Model file for the job. Use its own axes, mm. Round coordinates to 2 decimals unless told otherwise and drop trailing zeros. Write each loop counter-clockwise with the first axis right and the second up, starting at its lowest first coordinate (ties: lowest second). Pieces come first, ordered by that corner, then holes. Notation, with made-up numbers: (1, 69.5) - (13, 69.5) arc R23 ccw to (13, 102.5) - close; hole circle Ø1 at (-11, 43). An arc over 180 degrees is marked (long way). One line per item, written item: value.
Autodesk Inventor part; units mm, degrees
ref_plane "YZ Plane" through (0, 0, 0) normal (1, 0, 0) x (0, 1, 0)
ref_plane "XZ Plane" through (0, 0, 0) normal (0, 1, 0) x (-1, 0, 0)
ref_plane "XY Plane" through (0, 0, 0) normal (0, 0, 1) x (1, 0, 0)
sketch "Sketch1" plane through (0, 0, 0) normal (0, 1, 0) x (-1, 0, 0)
  line L0 (3.175, 0) -> (9.525, 0)
  line L1 (12.7, 3.175) -> (12.7, 200.025)
  line L2 (9.525, 203.2) -> (3.175, 203.2)
  line L3 (0, 200.025) -> (0, 3.175)
  circle A0 centre (6.35, 6.35) radius 2.5797
  circle A1 centre (6.35, 196.85) radius 2.5797
  circle A2 centre (6.35, 101.6) radius 2.5797
  arc A3 (12.7, 200.025) -> (9.525, 203.2) centre (9.525, 200.025) ccw
  arc A4 (3.175, 203.2) -> (0, 200.025) centre (3.175, 200.025) ccw
  arc A5 (0, 3.175) -> (3.175, 0) centre (3.175, 3.175) ccw
  arc A6 (9.525, 0) -> (12.7, 3.175) centre (9.525, 3.175) ccw
  point P0 (0, 0)
  point P1 (12.7, 0)
  point P2 (0, 203.2)
  dimension "d0" = 203.2
  dimension "d1" = 12.7
  dimension "d2" = 5.1594
  dimension "d3" = 6.35
  dimension "d4" = 6.35
  dimension "d5" = 5.1594
  dimension "d6" = 6.35
  dimension "d7" = 6.35
  dimension "d8" = 6.35
  dimension "d9" = 5.1594
  dimension "d10" = 101.6
  dimension "d11" = 3.175
extrude "Extrusion1" add sketch "Sketch1" along normal blind 9.525
fillet "Fillet1" radius 3.175 16 edges at (-0.9299, 9.525, 0.9299) (-6.35, 9.525, 0) (-11.7701, 9.525, 0.9299) (-12.7, 9.525, 101.6) (-11.7701, 9.525, 202.2701) (-6.35, 9.525, 203.2) (-0.9299, 9.525, 202.2701) (0, 9.525, 101.6) (-0.9299, 0, 0.9299) (-6.35, 0, 0) (-11.7701, 0, 0.9299) (-12.7, 0, 101.6) (-11.7701, 0, 202.2701) (-6.35, 0, 203.2) (-0.9299, 0, 202.2701) (0, 0, 101.6)
equation "\"d3\" = 0.5 * d1"
equation "\"d4\" = d3"
equation "\"d5\" = d2"
equation "\"d6\" = d4"
equation "\"d7\" = d6"
equation "\"d8\" = d7"
equation "\"d9\" = d5"
equation "\"d10\" = 0.5 * d0"
properties part number "Outer bar"
1. Drop flat-ended pins along their axis: pin 1 (1.5 mm diameter, centred on x = -11, z = 124, fed in from +Y); pin 2 (2 mm diameter, centred on x = -11, y = 2, fed in from -Z). Give the stop position or say it passes through.
Report:
pin 1: y = 9.44
pin 2: z = 0.13
2. Band-saw the part on D-D on y = 8. Write the cut outline in (x, z) (3 decimals).
Report:
outline: (-12.238, 3.175) arc R2.713 ccw to (-9.525, 0.462) - (-3.175, 0.462) arc R2.713 ccw to (-0.462, 3.175) - (-0.462, 200.025) arc R2.713 ccw to (-3.175, 202.738) - (-9.525, 202.738) arc R2.713 ccw to (-12.238, 200.025) - close; hole circle Ø5.159 at (-6.35, 6.35); hole circle Ø5.159 at (-6.35, 101.6); hole circle Ø5.159 at (-6.35, 196.85)
3. Band-saw the part on B-B on x = -6.35. Write the cut outline in (y, z) (3 decimals), plus the area to 3 significant figures.
Report:
outline: (0, 3.175) arc R3.175 ccw to (3.175, 0) - (6.35, 0) arc R3.175 ccw to (9.525, 3.175) - (9.525, 3.77) - (0, 3.77) - close; (0, 8.93) - (9.525, 8.93) - (9.525, 99.02) - (0, 99.02) - close; (0, 104.18) - (9.525, 104.18) - (9.525, 194.27) - (0, 194.27) - close; (0, 199.43) - (9.525, 199.43) - (9.525, 200.025) arc R3.175 ccw to (6.35, 203.2) - (3.175, 203.2) arc R3.175 ccw to (0, 200.025) - close
area: 1,780 mm²
4. Band-saw the part on C-C on z = 182.5. Write the cut outline in (x, y) (3 decimals), plus the area to 3 significant figures.
Report:
outline: (-12.7, 3.175) arc R3.175 ccw to (-9.525, 0) - (-3.175, 0) arc R3.175 ccw to (0, 3.175) - (0, 6.35) arc R3.175 ccw to (-3.175, 9.525) - (-9.525, 9.525) arc R3.175 ccw to (-12.7, 6.35) - close
area: 112 mm²
5. Band-saw the part on A-A on z = 6.35. Write the cut outline in (x, y) (3 decimals), plus the area to 3 significant figures.
Report:
outline: (-12.7, 3.175) arc R3.175 ccw to (-9.525, 0) - (-8.93, 0) - (-8.93, 9.525) - (-9.525, 9.525) arc R3.175 ccw to (-12.7, 6.35) - close; (-3.77, 0) - (-3.175, 0) arc R3.175 ccw to (0, 3.175) - (0, 6.35) arc R3.175 ccw to (-3.175, 9.525) - (-3.77, 9.525) - close
area: 63.2 mm²
6. Mould opens along X. For faces 1 (the face through (-0.91, 4.74, 202.25)), 2 (the face through (-6.306, 8.62, 202.245)), 3 (the face through (-6.014, 4.696, 194.292)) say: released by +X, released by -X, zero draft, split by the parting line, or undercut.
Report:
face 1: released by +X
face 2: zero draft
face 3: undercut
7. Wall check: probe 1 along Z at (x, y) = (-6.35, 3); probe 2 along X at (y, z) = (4.25, 196.85); probe 3 along Z at (x, y) = (-6.35, 2.5). Give the ranges that are in metal, low to high. Write a range as [from, to].
Report:
probe 1: [0, 3.77], [8.93, 99.02], [104.18, 194.27], [199.43, 203.2]
probe 2: [-12.7, -8.93], [-3.77, 0]
probe 3: [0.07, 3.77], [8.93, 99.02], [104.18, 194.27], [199.43, 203.13]
